from build123d import *

# Parameters (mm, degrees)
SKETCH_1_W          = 70
SKETCH_1_H          = 74
EXTRUDE_1_DEPTH     = 5
CUT_EXTRUDE_2_REACH = 103.985
SKETCH_2_W          = 60
SKETCH_2_H          = 2.2
SKETCH_3_W          = 56.4
SKETCH_3_H          = 56.4
CUT_EXTRUDE_3_DEPTH = 20
SKETCH_4_W          = 3.6
SKETCH_4_H          = 61.4
CUT_EXTRUDE_5_DEPTH = 102.985293057
SKETCH_5_R          = 6.5
EXTRUDE_6_DEPTH     = 5
CUT_EXTRUDE_7_REACH = 103.985
SKETCH_6_R          = 1.9


with BuildPart() as part:
    # Эскиз1 → Вытянуть1 (new body)
    with BuildSketch(Plane.XY):
        with Locations((35, 37)):
            Rectangle(SKETCH_1_W, SKETCH_1_H)
    extrude(amount=EXTRUDE_1_DEPTH)

    # Эскиз2 → Вытянуть2 (cut, up to next)
    with BuildSketch(Plane.XY.offset(5), mode=Mode.PRIVATE) as cut_extrude_2_sk1:
        with Locations((35, 6.1)):
            Rectangle(SKETCH_2_W, SKETCH_2_H)
    cut_extrude_2_tool1 = extrude(cut_extrude_2_sk1.sketch, amount=-CUT_EXTRUDE_2_REACH, mode=Mode.PRIVATE) & part.part
    add(cut_extrude_2_tool1.solids().sort_by_distance((35, 6.1, 5))[0], mode=Mode.SUBTRACT)

    # Эскиз3 → Вытянуть3 (cut)
    with BuildSketch(Plane.XY.offset(5)):
        with Locations((33.2, 40.8)):
            Rectangle(SKETCH_3_W, SKETCH_3_H)
    extrude(amount=-CUT_EXTRUDE_3_DEPTH, mode=Mode.SUBTRACT)

    # Эскиз4 → Вытянуть5 (cut, through all)
    with BuildSketch(Plane(origin=(0, 0, 0), x_dir=(-1, 0, 0), z_dir=(0, 0, -1))):
        with Locations((-68.2, 43.3)):
            Rectangle(SKETCH_4_W, SKETCH_4_H)
    extrude(amount=-CUT_EXTRUDE_5_DEPTH, mode=Mode.SUBTRACT)

    # Эскиз5 → Вытянуть6 (add)
    with BuildSketch(Plane.XY.offset(5)):
        with Locations((-1.5, 23.329095616)):
            Circle(SKETCH_5_R)
    extrude(amount=-EXTRUDE_6_DEPTH)

    # Эскиз6 → Вытянуть7 (cut, up to next)
    with BuildSketch(Plane.XY.offset(5), mode=Mode.PRIVATE) as cut_extrude_7_sk1:
        with Locations((-1.5, 23.329095616)):
            Circle(SKETCH_6_R)
    cut_extrude_7_tool1 = extrude(cut_extrude_7_sk1.sketch, amount=-CUT_EXTRUDE_7_REACH, mode=Mode.PRIVATE) & part.part
    add(cut_extrude_7_tool1.solids().sort_by_distance((-1.5, 23.329096, 5))[0], mode=Mode.SUBTRACT)


solid = part.part
The model under review builds one solid part; all positions refer to its coordinate system, in mm. A direction names the side the tool comes from. Round coordinates to 2 decimals unless told otherwise and drop trailing zeros. Loops run counter-clockwise (first coordinate to the right, second up) from the corner with the lowest first, then second, coordinate; pieces in that order, holes last. Notation, with made-up numbers: M 8,88 L 51,88 A15 ccw 51,112 Z; hole C 52.5,81.5 d11. An arc over 180 degrees is marked long. Answer as a JSON object with one key per item and string values.
Item 1: We need section B-B, the plane x = -1.5. State the section outline as (y, z) points, and give its area (3 significant figures).
Check sheet entries:
{"outline": "M 16.83,0 L 21.43,0 L 21.43,5 L 16.83,5 Z; M 25.23,0 L 29.83,0 L 29.83,5 L 25.23,5 Z", "area": "46.0 mm2"}
Item 2: We need section D-D, the plane x = 48. State the section outline as (y, z) points.
Check sheet entries:
{"outline": "M 0,0 L 5,0 L 5,5 L 0,5 Z; M 7.2,0 L 12.6,0 L 12.6,5 L 7.2,5 Z; M 69,0 L 74,0 L 74,5 L 69,5 Z"}
Item 3: Clearance check with flat-ended pins moving along their axes: P1, Ø1.5, axis at y = 46, z = 3, coming from the +X side; P2, Ø1.5, axis at x = 26, z = 2.5, coming from the -Y side; P3, Ø1.1, axis at x = 67.5, z = 1.5, coming from the +Y side; P4, Ø2.5, axis at y = 4.5, z = 1.5, coming from the -X side. State where each tip first meets the part, or that it passes through.
Check sheet entries:
{"P1": "x = 66.4", "P2": "y = 0", "P3": "y = 12.6", "P4": "x = 0"}
Item 4: The part is to be moulded in two halves that separate along Y. For faces 4 (the face through (70, 6, 2)), 5 (the face through (35, 0, 2)), 6 (the face through (65, 6, 3)), say which applies: +Y half, -Y half, draft (parallel to the pull), parting line (faces both ways), or undercut.
Check sheet entries:
{"face 4": "draft", "face 5": "-Y half", "face 6": "undercut"}
Item 5: We need section C-C, the plane z = 2.2. State the section outline as (x, y) points.
Check sheet entries:
{"outline": "M 0,0 L 70,0 L 70,12.6 L 66.4,12.6 L 66.4,74 L 0,74 L 0,29.65 A6.5 ccw long 0,17 Z; hole C -1.5,23.33 d3.8; hole M 5,5 L 65,5 L 65,7.2 L 5,7.2 Z; hole M 5,12.6 L 61.4,12.6 L 61.4,69 L 5,69 Z"}
Item 6: We need section A-A, the plane y = 36. State the section outline as (x, z) points, and give its area (3 significant figures).
Check sheet entries:
{"outline": "M 0,0 L 5,0 L 5,5 L 0,5 Z; M 61.4,0 L 66.4,0 L 66.4,5 L 61.4,5 Z", "area": "50.0 mm2"}
Item 7: Tool access review of faces 1 (the face through (66.4, 43, 2)), 2 (the face through (4, 38, 0)), 3 (the face through (5, 40, 3)): name each direction out of +Z, -Z, +X, -X, +Y, -Y from which nothing blocks a thin tool from reaching the whole face with its end or side.
Check sheet entries:
{"face 1": "+Z, -Z, +X, +Y", "face 2": "-Z, +X, -X, +Y, -Y", "face 3": "+Z, -Z"}
Item 8: For line 1 along Y through (x, z) = (12.5, 1.45); line 2 along Y through (x, z) = (-1.5, 3.15); line 3 along X through (y, z) = (50, 0.5), list the stretches that pass through material, from the lowest coordinate up.
Check sheet entries:
{"line 1": "0 to 5, 7.2 to 12.6, 69 to 74", "line 2": "16.83 to 21.43, 25.23 to 29.83", "line 3": "0 to 5, 61.4 to 66.4"}
